Verification items for the finished model (mm, model axes). A direction names the side the tool comes from. Give positions to 0.01 mm unless a question says otherwise; leave off trailing zeros. Order: outer loops, then holes, each group sorted by start corner. A loop starts at its lowest first (then second) coordinate and runs counter-clockwise, first axis right, second up. Notation, with made-up numbers: (17.25, 24.5) -> (61.25, 24.5) arc R11 cw to (61.25, 32.5) -> close; hole circle Ø8 at (4.5, 64). An arc over 180 degrees is marked (long way). Return JSON: item names as keys, results as strings. Group by question number.
(1) Cross-section at A-A on x = 140. Enter the section's corners in (y, z) (3 decimals).
(2) Cross-section at B-B on z = 1.55. State how many separate pieces and enclosed holes the cut face has, then the cut area to 3 significant figures.
(3) Release check for a two-part mould opening along Y. For faces 1 (the face through (162, 45.72, 3)), 2 (the face through (90.519, 199, 3)), 3 (the face through (275, 22.86, 3)), 4 (the face through (176, 195.72, 3)) record: pulls with the +Y half, pulls with the -Y half, needs draft (parallel to the pull), parting line crosses it, or undercut.
(4) Tool access check on faces 5 (the face through (150, 34.29, 3)), 6 (the face through (204.819, 199, 3)), 7 (the face through (291.83, 31, 3)), 8 (the face through (140, 45.72, 3)). Record the directions out of +Z, -Z, +X, -X, +Y, -Y that give a thin tool (end or side, any length) a straight path to the whole face; none if there is none.
(5) Cross-section at D-D on x = 229.5. Enter the section's corners in (y, z) (3 decimals).
(6) Cross-section at C-C on y = 76. Enter the section's corners in (x, z) (3 decimals), then the cut area to 3 significant figures.
(7) Thickness scan on line 1 along Y through (x, z) = (112, 3.15); line 2 along Y through (x, z) = (164, 4.95); line 3 along Y through (x, z) = (60.5, 0.2). Record the ranges inside material, lowest first.
(8) Depth check by flat-ended pin: pin 1 Ø10 at (x, y) = (233, 49.5) entering from -Z; pin 2 Ø1.7 at (y, z) = (197, 4) entering from -X; pin 3 Ø1.7 at (x, z) = (137.5, 3) entering from -Y; pin 4 Ø1.7 at (y, z) = (41.5, 3) entering from +X. Enter the tip coordinate at first touch or a pass-through.
from build123d import *

# Parameters (mm, degrees)
BOSS_EXTRUDE1_DEPTH = 5.715


with BuildPart() as part:
    # Model → Boss-Extrude1 (new body)
    with BuildSketch(Plane.XY):
        Polygon((16.115014462, 22.860238699), (38.975005129, 22.860238699), (41.932961262, 23.249623789), (44.690011654, 24.391232573), (47.057297821, 26.208001576), (48.873953439, 28.575245224), (50.690254725, 30.942499501), (53.057186561, 32.759257875), (55.814102307, 33.900880832), (58.772193086, 34.290251749), (243.45807324, 34.290251749), (246.416029373, 33.900880832), (249.173079765, 32.759257875), (251.539834435, 30.942499501), (253.355958556, 28.575245224), (255.172925985, 26.208001576), (257.540254672, 24.391232573), (260.297170418, 23.249623789), (263.255261197, 22.860238699), (286.114932966, 22.860238699), (286.114932966, 25.834246031), (291.829939491, 25.834246031), (291.829939491, 37.264294514), (286.114932966, 37.264294514), (286.114932966, 48.694307564), (291.829939491, 48.694307564), (291.829939491, 60.124320614), (286.114932966, 60.124320614), (286.114932966, 71.554333664), (291.829939491, 71.554333664), (291.829939491, 82.984346714), (286.114932966, 82.984346714), (286.114932966, 94.414359764), (291.829939491, 94.414359764), (291.829939491, 105.844372814), (286.114932966, 105.844372814), (286.114932966, 117.274385864), (291.829939491, 117.274385864), (291.829939491, 128.704398914), (286.114932966, 128.704398914), (286.114932966, 131.679362941), (286.114932966, 135.720154956), (276.321220997, 145.514221256), (280.362013012, 149.556430596), (272.279011657, 157.638368957), (268.238219642, 153.597222611), (260.15592695, 161.679160972), (264.197073296, 165.720307318), (256.115134935, 173.80224568), (252.073988588, 169.761453665), (243.992050227, 177.843392026), (248.033196573, 181.884184041), (239.951258212, 189.967185396), (235.909048873, 185.926393381), (226.114982572, 195.720459681), (222.074190557, 195.720459681), (216.248987056, 195.720459681), (216.248987056, 201.435466206), (204.818974006, 201.435466206), (204.818974006, 195.720459681), (193.388960956, 195.720459681), (193.388960956, 201.435466206), (181.958947906, 201.435466206), (181.958947906, 195.720459681), (170.528934856, 195.720459681), (170.528934856, 201.435466206), (159.098921806, 201.435466206), (159.098921806, 195.720459681), (147.668908756, 195.720459681), (147.668908756, 201.435466206), (136.238895706, 201.435466206), (136.238895706, 195.720459681), (124.808882656, 195.720459681), (124.808882656, 201.435466206), (113.378869606, 201.435466206), (113.378869606, 195.720459681), (101.949210887, 195.720459681), (101.949210887, 201.435466206), (90.519197837, 201.435466206), (90.519197837, 195.720459681), (79.089184787, 195.720459681), (79.089184787, 201.435466206), (67.659171737, 201.435466206), (67.659171737, 195.720459681), (56.229158687, 195.720459681), (56.229158687, 201.435466206), (44.799145637, 201.435466206), (44.799145637, 195.720459681), (33.369026287, 195.720459681), (33.369026287, 201.435466206), (21.939013237, 201.435466206), (21.939013237, 195.720459681), (16.115014462, 195.720459681), (16.115014462, 183.585327716), (10.400007937, 183.585327716), (10.400007937, 172.155314666), (16.115014462, 172.155314666), (16.115014462, 160.725301616), (10.400007937, 160.725301616), (10.400007937, 149.295288565), (16.115014462, 149.295288565), (16.115014462, 137.865275515), (10.400007937, 137.865275515), (10.400007937, 126.435262465), (16.115014462, 126.435262465), (16.115014462, 115.005249415), (10.400007937, 115.005249415), (10.400007937, 103.575236365), (16.115014462, 103.575236365), (16.115014462, 92.145223315), (10.400007937, 92.145223315), (10.400007937, 80.715210265), (16.115014462, 80.715210265), (16.115014462, 69.285197215), (10.400007937, 69.285197215), (10.400007937, 57.855184165), (16.115014462, 57.855184165), (16.115014462, 46.425171115), (10.400007937, 46.425171115), (10.400007937, 34.995264365), (16.115014462, 34.995264365), align=None)
        Polygon((25.385025046, 40.005400006), (19.670018521, 40.005400006), (19.670018521, 45.720406531), (31.099996138, 45.720406531), (31.099996138, 40.005400006), align=None, mode=Mode.SUBTRACT)
        Polygon((48.245015713, 40.005400006), (42.530009188, 40.005400006), (42.530009188, 45.720406531), (53.960022238, 45.720406531), (53.960022238, 40.005400006), align=None, mode=Mode.SUBTRACT)
        Polygon((71.105041813, 40.005400006), (65.390035288, 40.005400006), (65.390035288, 45.720406531), (76.820048338, 45.720406531), (76.820048338, 40.005400006), align=None, mode=Mode.SUBTRACT)
        Polygon((93.965067913, 40.005400006), (88.250061388, 40.005400006), (88.250061388, 45.720406531), (99.680074438, 45.720406531), (99.680074438, 40.005400006), align=None, mode=Mode.SUBTRACT)
        Polygon((116.825094013, 40.005400006), (111.110087488, 40.005400006), (111.110087488, 45.720406531), (122.540100538, 45.720406531), (122.540100538, 40.005400006), align=None, mode=Mode.SUBTRACT)
        Polygon((139.685120113, 40.005400006), (133.970113588, 40.005400006), (133.970113588, 45.720406531), (145.400126638, 45.720406531), (145.400126638, 40.005400006), align=None, mode=Mode.SUBTRACT)
        Polygon((162.545146213, 40.005400006), (156.830139688, 40.005400006), (156.830139688, 45.720406531), (168.260152738, 45.720406531), (168.260152738, 40.005400006), align=None, mode=Mode.SUBTRACT)
        Polygon((185.405172313, 40.005400006), (179.690165788, 40.005400006), (179.690165788, 45.720406531), (191.120178838, 45.720406531), (191.120178838, 40.005400006), align=None, mode=Mode.SUBTRACT)
        Polygon((208.265198413, 40.005400006), (202.550191888, 40.005400006), (202.550191888, 45.720406531), (213.980204938, 45.720406531), (213.980204938, 40.005400006), align=None, mode=Mode.SUBTRACT)
        Polygon((231.125224513, 40.005400006), (225.410217988, 40.005400006), (225.410217988, 45.720406531), (236.840231038, 45.720406531), (236.840231038, 40.005400006), align=None, mode=Mode.SUBTRACT)
        Polygon((253.985250613, 40.005400006), (248.270244088, 40.005400006), (248.270244088, 45.720406531), (259.700257138, 45.720406531), (259.700257138, 40.005400006), align=None, mode=Mode.SUBTRACT)
        Polygon((276.844922382, 40.005400006), (271.130270188, 40.005400006), (271.130270188, 45.720406531), (282.559928907, 45.720406531), (282.559928907, 40.005400006), align=None, mode=Mode.SUBTRACT)
    extrude(amount=BOSS_EXTRUDE1_DEPTH)


solid = part.part
Verdict:
{
 "1": {"outline": "(34.29, 0) -> (40.005, 0) -> (40.005, 5.715) -> (34.29, 5.715) -> close; (45.72, 0) -> (201.435, 0) -> (201.435, 5.715) -> (45.72, 5.715) -> close"},
 "2": {"separate pieces": "1", "enclosed holes": "12", "area": "43,300 mm²"},
 "3": {"face 1": "undercut", "face 2": "needs draft", "face 3": "pulls with the -Y half", "face 4": "pulls with the +Y half"},
 "4": {"face 5": "+Z, -Z, -Y", "face 6": "+Z, -Z, +Y", "face 7": "+Z, -Z, +X, +Y, -Y", "face 8": "+Z, -Z"},
 "5": {"outline": "(34.29, 0) -> (40.005, 0) -> (40.005, 5.715) -> (34.29, 5.715) -> close; (45.72, 0) -> (192.335, 0) -> (192.335, 5.715) -> (45.72, 5.715) -> close"},
 "6": {"outline": "(16.115, 0) -> (291.83, 0) -> (291.83, 5.715) -> (16.115, 5.715) -> close", "area": "1,580 mm²"},
 "7": {"line 1": "34.29 to 40.01, 45.72 to 195.72", "line 2": "34.29 to 40.01, 45.72 to 201.44", "line 3": "34.29 to 195.72"},
 "8": {"pin 1": "z = 0", "pin 2": "x = 21.94", "pin 3": "y = 34.29", "pin 4": "x = 286.11"}
}
